```python
from build123d import *

# Parameters (mm, degrees)
F0_R     = 101.6
F1_DEPTH = 127


with BuildPart() as f1:
    # F0 (on Front) → F1 (new body)
    with BuildSketch(Plane.XZ):
        with BuildLine():
            ThreePointArc((-722.9421635172, -249.79241048), (-548.1645057738, -175.6208384233), (-476.0120778236, 0))
            ThreePointArc((-476.0120778236, 0), (-545.3928207836, 172.7720479201), (-714.9961059612, 249.5743505755))
            ThreePointArc((-714.9961059612, 249.5743505755), (-975.5365160272, 6.8364028409), (-728.6671666698, -249.7927866438))
            Line((-728.6671666698, -249.7927866438), (-722.9421635172, -249.79241048))
        make_face()
        with Locations((-725.5384325981, 0)):
            Circle(F0_R, mode=Mode.SUBTRACT)
        with BuildLine():
            ThreePointArc((-714.9961059612, 249.5743505755), (-545.3928207836, 172.7720479201), (-476.0120778236, 0))
            Line((-476.0120778236, 0), (546.179202095, 0))
            ThreePointArc((546.179202095, 0), (617.2275203446, 174.4968628404), (789.9586907535, 249.7362237922))
            Line((789.9586907535, 249.7362237922), (-714.9961059612, 249.5743505755))
        make_face()
        with BuildLine():
            Line((546.179202095, 0), (-476.0120778236, 0))
            ThreePointArc((-476.0120778236, 0), (-548.1645057738, -175.6208384233), (-722.9421635172, -249.79241048))
            Line((-722.9421635172, -249.79241048), (788.379779932, -249.6931084215))
            ThreePointArc((788.379779932, -249.6931084215), (616.6767568201, -173.9308542911), (546.179202095, 0))
        make_face()
        with BuildLine():
            ThreePointArc((789.9586907535, 249.7362237922), (617.2275203446, 174.4968628404), (546.179202095, 0))
            ThreePointArc((546.179202095, 0), (616.6767568201, -173.9308542911), (788.379779932, -249.6931084215))
            Line((788.379779932, -249.6931084215), (803.6294365785, -249.6921064362))
            ThreePointArc((803.6294365785, -249.6921064362), (975.3110751844, -173.91907218), (1045.797202095, 0))
            ThreePointArc((1045.797202095, 0), (970.4850649354, 178.7606817504), (789.9586907535, 249.7362237922))
        make_face()
        with BuildLine():
            ThreePointArc((899.1158691406, 0), (797.5158691406, -101.6), (695.9158691406, 0))
            ThreePointArc((695.9158691406, 0), (797.5158691406, 101.6), (899.1158691406, 0))
        make_face(mode=Mode.SUBTRACT)
        with BuildLine():
            ThreePointArc((-728.6671666698, -249.7927866438), (-725.8046640158, -249.8089994608), (-722.9421635172, -249.79241048))
            Line((-722.9421635172, -249.79241048), (-728.6671666698, -249.7927866438))
        make_face()
        with BuildLine():
            Line((803.6294365785, -249.6921064362), (788.379779932, -249.6931084215))
            ThreePointArc((788.379779932, -249.6931084215), (796.0046159028, -249.8089994608), (803.6294365785, -249.6921064362))
        make_face()
    extrude(amount=F1_DEPTH)


solid = f1.part
```
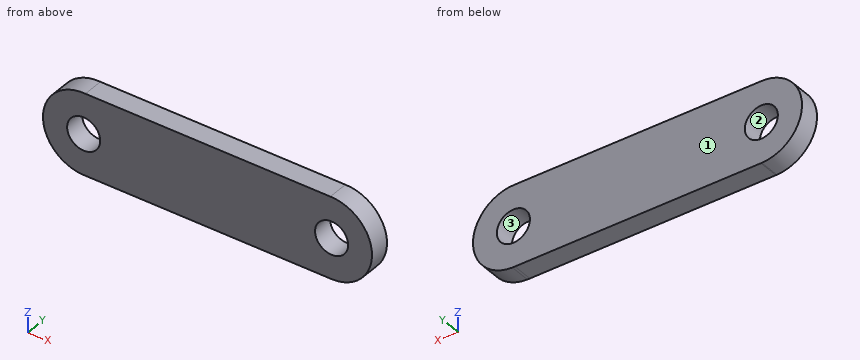
CAD build for the part. Positions are in the model's coordinates, mm. Face numbers are marked on the shaded views. Coordinates: 2 decimals unless noted, no trailing zeros. Order: outer loops, then holes, each group sorted by start corner. A loop starts at its lowest first (then second) coordinate and runs counter-clockwise, first axis right, second up. Notation, with made-up numbers: (-8.5, 75) - (4.5, 75) arc R26 ccw to (4.5, 100) - close; hole circle Ø2 at (85, 66). An arc over 180 degrees is marked (long way). Use a Markdown table: item, result. Add a question column.
(1) Saw through at D-D (x = -806). Give the cut face in (y, z).
(2) Saw through at B-B (y = -25). Give the cut face in (x, z).
(3) Pull direction X, two halves, no side cores. Call the marked faces 1, 2 and 3: +X half, -X half, draft (parallel to the pull), parting line (faces both ways), or undercut.
(4) Drill centre lines: line 1 along X through (y, z) = (-87, 3); line 2 along X through (y, z) = (-89.5, -47); line 3 along Z through (x, y) = (543, -69). Where is each one in solid material? Low to high. Write a range as [from, to].
(5) Flat gauge pins, fed straight in: pin 1 (12 mm diameter, centred on y = -24.5, z = 13.5, fed in from -X); pin 2 (1 mm diameter, centred on y = -94, z = -166, fed in from +X); pin 3 (4 mm diameter, centred on y = -73.5, z = 177.5, fed in from -X). Where does each tip first touch, or does it go through?
(6) Saw through at C-C (x = 878). Give the cut face in (y, z), then the cut area to 3 significant figures.
(7) Saw through at A-A (z = 0). Give the cut face in (x, y).
Solved:
| question | item | result |
|---|---|---|
| 1 | outline | (-127, -236.59) - (0, -236.59) - (0, -62.04) - (-127, -62.04) - close; (-127, 62.04) - (0, 62.04) - (0, 236.59) - (-127, 236.59) - close |
| 2 | outline | (-722.94, -249.79) - (788.38, -249.69) arc R249.81 ccw (long way) to (789.96, 249.74) - (-715, 249.57) arc R249.81 ccw (long way) to start; hole circle Ø203.2 at (-725.54, 0); hole circle Ø203.2 at (797.52, 0) |
| 3 | face 1 | draft |
| 3 | face 2 | undercut |
| 3 | face 3 | undercut |
| 4 | line 1 | x = [-975.61, -827.09], [-623.98, 695.96], [899.07, 1045.78] |
| 4 | line 2 | x = [-971.17, -815.61], [-635.46, 707.44], [887.59, 1041.34] |
| 4 | line 3 | z = [-249.71, 249.71] |
| 5 | pin 1 | stops at x = -975.52 |
| 5 | pin 2 | stops at x = 983.11 |
| 5 | pin 3 | stops at x = -903.6 |
| 6 | outline | (-127, -235.96) - (0, -235.96) - (0, -62.01) - (-127, -62.01) - close; (-127, 62.01) - (0, 62.01) - (0, 235.96) - (-127, 235.96) - close |
| 6 | area | 44,200 mm² |
| 7 | outline | (-975.63, -127) - (-827.14, -127) - (-827.14, 0) - (-975.63, 0) - close; (-623.94, -127) - (695.92, -127) - (695.92, 0) - (-623.94, 0) - close; (899.12, -127) - (1045.8, -127) - (1045.8, 0) - (899.12, 0) - close |
